Work out the finished part from the listing and answer in its coordinate system (mm). A direction names the side the tool comes from. Round coordinates to 2 decimals unless told otherwise and drop trailing zeros. Loops run counter-clockwise (first coordinate to the right, second up) from the corner with the lowest first, then second, coordinate; pieces in that order, holes last.
Autodesk Fusion 360 part; units mm, degrees
sketch "Sketch1" plane through (0, 0, 0) normal (0, 0, 1) x (1, 0, 0)
  line L0 (-75, 75) -> (75, 75)
  line L1 (75, 75) -> (75, -25)
  line L2 (75, -25) -> (-75, -25)
  line L3 (-75, -25) -> (-75, 75)
  dimension "d1" = 150
  dimension "d2" = 100
extrude "Extrude1" add sketch "Sketch1" along normal blind 10
sketch "Sketch2" plane through (0, 0, 10) normal (0, 0, 1) x (-1, 0, 0)
  line L0 (75, 25) -> (-75, 25)
  line L1 (-75, 25) -> (-75, -75)
  line L2 (-75, -75) -> (75, -75)
  line L3 (75, -75) -> (75, 25)
  line L4 (-75, 25) -> (75, 25)
  line L5 (75, 25) -> (75, 0)
  line L6 (75, 0) -> (-75, 0)
  line L7 (-75, 0) -> (-75, 25)
extrude "Extrude2" add sketch "Sketch2" along normal blind 75 contours L0 L1 L3 L4 L5 L6 L7
sketch "Sketch3" plane through (0, 0, 10) normal (0, 0, 1) x (-1, 0, 0)
  line L0 (75, 0) -> (-75, 0)
  line L1 (-75, 0) -> (-75, -75)
  line L2 (-75, -75) -> (75, -75)
  line L3 (75, -75) -> (75, 0)
extrude "Extrude3" add sketch "Sketch3" along normal blind 5
extrude "Extrude4" add 1 faces at (25, 75, 5) along direction (0, 1, 0) blind 20
sketch "Sketch4" plane through (0, 0, 15) normal (0, 0, 1) x (-1, 0, 0)
  line L0 (75, -95) -> (75, 0)
  line L1 (75, 0) -> (-75, 0)
  line L2 (-75, 0) -> (-75, -95)
  line L3 (-75, -95) -> (75, -95)
  line L4 (-75, -75) -> (75, -75)
  line L5 (75, -75) -> (75, -95)
  line L6 (75, -95) -> (-75, -95)
  line L7 (-75, -95) -> (-75, -75)
extrude "Extrude5" add sketch "Sketch4" along normal blind 50 contours L0 L2 L3 L4 L5 L6 L7
fillet "Fillet1" radius 15 1 edges at (0, 0, 15)
fillet "Fillet2" radius 15 1 edges at (0, 75, 15)
sketch "Sketch5" plane through (0, 0, 85) normal (0, 0, 1) x (-1, 0, 0)
  line L0 (-75, 0) -> (75, 0)
  line L1 (75, 0) -> (75, 25)
  line L2 (75, 25) -> (-75, 25)
  line L3 (-75, 25) -> (-75, 0)
  line L4 (65, 10) -> (50, 10)
  line L5 (50, 10) -> (50, 15)
  line L6 (50, 15) -> (65, 15)
  line L7 (65, 15) -> (65, 10)
  line L8 (35, 10) -> (20, 10)
  line L9 (20, 10) -> (20, 15)
  line L10 (20, 15) -> (35, 15)
  line L11 (35, 15) -> (35, 10)
  line L12 (5, 10) -> (-10, 10)
  line L13 (-10, 10) -> (-10, 15)
  line L14 (-10, 15) -> (5, 15)
  line L15 (5, 15) -> (5, 10)
  line L16 (-25, 10) -> (-40, 10)
  line L17 (-40, 10) -> (-40, 15)
  line L18 (-40, 15) -> (-25, 15)
  line L19 (-25, 15) -> (-25, 10)
  line L20 (-50, 10) -> (-65, 10)
  line L21 (-65, 10) -> (-65, 15)
  line L22 (-65, 15) -> (-50, 15)
  line L23 (-50, 15) -> (-50, 10)
extrude "Extrude6" add sketch "Sketch5" along normal blind 5 contours L4 L5 L6 L7 | L8 L9 L10 L11 | L12 L13 L14 L15 | L16 L17 L18 L19 | L20 L21 L22 L23
fillet "Fillet3" radius 10 1 faces at (-25, 88.3333, 65)
extrude "Extrude7" cut 1 faces at (0, -11.6667, 90) along direction (0, 0, -1) blind 10
extrude "Extrude8" cut 1 faces at (-30, -11.6667, 90) along direction (0, 0, -1) blind 10
extrude "Extrude9" cut 1 faces at (-60, -11.6667, 90) along direction (0, 0, -1) blind 10
extrude "Extrude10" cut 1 faces at (30, -11.6667, 90) along direction (0, 0, -1) blind 10
extrude "Extrude11" cut 1 faces at (55, -11.6667, 90) along direction (0, 0, -1) blind 10
1. Given pin 1 (5.5 mm diameter, centred on x = -27, y = -12.5, fed in from +Z); pin 2 (5.5 mm diameter, centred on x = 32.5, z = 83, fed in from +Y); pin 3 (1.5 mm diameter, centred on x = 33.5, y = -12, fed in from +Z); pin 4 (2 mm diameter, centred on x = 43, y = 38.5, fed in from +Z), each flat-ended and moving along its own axis, determine where each tip first touches the part or whether it passes through.
Answer key:
pin 1: stops at z = 85
pin 2: stops at y = 0
pin 3: stops at z = 80
pin 4: stops at z = 15
2. Find section C-C (y = 78). Write down the section's boundary in (x, z).
Answer key:
outline: (-75, 0) - (75, 0) - (75, 55) arc R10 ccw to (72, 62.14) - (-72, 62.14) arc R10 ccw to (-75, 55) - close
3. Which of the six approach directions +Z, -Z, +X, -X, +Y, -Y give full straight-line access (tool end or side, diameter ignored) to faces 1 (the face through (1, 95, 27)), 2 (the face through (40, -12, 83)), 3 (the face through (1, 75, 42))?
Answer key:
face 1: +Z, -Z, +X, -X, +Y
face 2: +Z
face 3: +Z, +X, -X
4. Find section D-D (z = 67). Write down the section's boundary in (x, y), then the cut area to 3 significant figures.
Answer key:
outline: (-75, -25) - (75, -25) - (75, 0) - (-75, 0) - close
area: 3,750 mm2
5. Find section A-A (z = 38.5). Write down the section's boundary in (x, y).
Answer key:
outline: (-75, -25) - (75, -25) - (75, 0) - (-75, 0) - close; (-75, 75) - (75, 75) - (75, 95) - (-75, 95) - close
6. Determine the mould class of faces 4 (the face through (-1.05, 91.99, 62.15)), 5 (the face through (73, 85, 61)), 6 (the face through (57, -10, 83)) for opening direction X: +X half, -X half, draft (parallel to the pull), parting line (faces both ways), or undercut.
Answer key:
face 4: draft
face 5: +X half
face 6: undercut
7. Consider probe 1 along Y at (x, z) = (-56, 39.5); probe 2 along Y at (x, z) = (-57, 81); probe 3 along Z at (x, y) = (64, 39.5). Determine where each line is inside the solid, lowest interval first.
Answer key:
probe 1: y = -25 to 0, 75 to 95
probe 2: y = -25 to -15, -10 to 0
probe 3: z = 0 to 15
